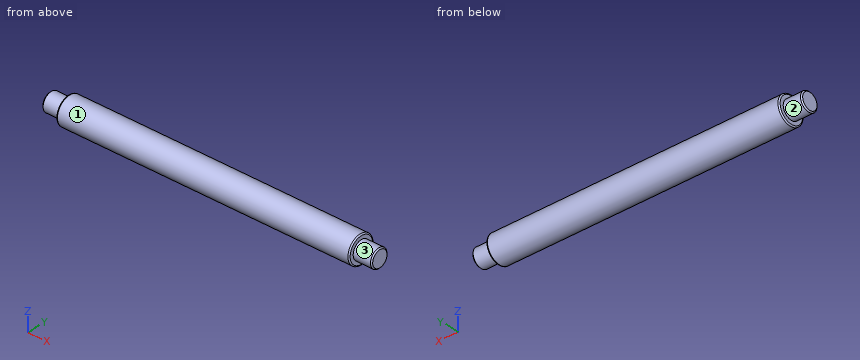
```python
from build123d import *

# Parameters (mm, degrees)
CHAMFER3_SIZE = 0.25
FILLET1_R     = 0.25


with BuildPart() as part:
    # Sketch1 → Revolve1 (revolve)
    with BuildSketch(Plane.XY, mode=Mode.PRIVATE) as revolve1_sk:
        Polygon((-35.75, 0), (-35.75, 2), (-31.75, 2), (-31.75, 3), (31.75, 3), (31.75, 2), (35.75, 2), (35.75, 0), align=None)
    revolve(revolve1_sk.sketch.rotate(Axis((-39.77575721, 0, 0), (1, 0, 0)), 90), axis=Axis((-39.77575721, 0, 0), (1, 0, 0)))

    # Chamfer3
    chamfer3_edges = [part.edges().sort_by_distance(p)[0] for p in [
        (35.75, 0, -2),
        (-35.75, 0, -2),
    ]]
    chamfer(chamfer3_edges, length=CHAMFER3_SIZE)

    # Fillet1
    fillet1_edges = [part.edges().sort_by_distance(p)[0] for p in [
        (31.75, 0, -3),
        (-31.75, 0, -3),
    ]]
    fillet(fillet1_edges, radius=FILLET1_R)


solid = part.part
```
Here's how the part is built. I have some questions about the finished solid (model axes, mm). Face numbers are marked on the shaded views. A direction names the side the tool comes from. Round coordinates to 2 decimals unless told otherwise and drop trailing zeros. Loops run counter-clockwise (first coordinate to the right, second up) from the corner with the lowest first, then second, coordinate; pieces in that order, holes last.
1. Will these pins go through, and if not, where does the flat tip stop? pin 1 (2 mm diameter, centred on x = -16.5, z = -2, fed in from -Y); pin 2 (1 mm diameter, centred on y = -2.5, z = -0.5, fed in from +X); pin 3 (1.5 mm diameter, centred on x = -17, y = 2.5, fed in from +Z).
Answers:
pin 1: stops at y = -2.83
pin 2: stops at x = 31.75
pin 3: stops at z = 2.44
2. Suppose I cut it at A-A, the plane z = 0. Please give me the cut outline in (x, y), and give its area (3 significant figures).
Answers:
outline: (-35.75, -1.75) - (-35.5, -2) - (-31.75, -2) - (-31.75, -2.75) arc R0.25 ccw to (-31.5, -3) - (31.5, -3) arc R0.25 ccw to (31.75, -2.75) - (31.75, -2) - (35.5, -2) - (35.75, -1.75) - (35.75, 1.75) - (35.5, 2) - (31.75, 2) - (31.75, 2.75) arc R0.25 ccw to (31.5, 3) - (-31.5, 3) arc R0.25 ccw to (-31.75, 2.75) - (-31.75, 2) - (-35.5, 2) - (-35.75, 1.75) - close
area: 413 mm2
3. For the marked faces 1, 2 and 3, which set-ups out of +Z, -Z, +X, -X, +Y, -Y let a thin tool reach every point of the face, with its end or its side?
Answers:
face 1: +X, -X
face 2: -X
face 3: +X
4. If I drill on probe 1 along X at (y, z) = (-2, 1.25); probe 2 along Z at (x, y) = (-13.5, -0.25); probe 3 along Z at (x, y) = (14, 1.5), over which ranges is the centre line in solid material (lowest first)?
Answers:
probe 1: x = -31.75 to 31.75
probe 2: z = -2.99 to 2.99
probe 3: z = -2.6 to 2.6
5. Suppose I cut it at C-C, the plane x = -5. Please give me the cut outline in (y, z).
Answers:
outline: circle Ø6 at (0, 0)
